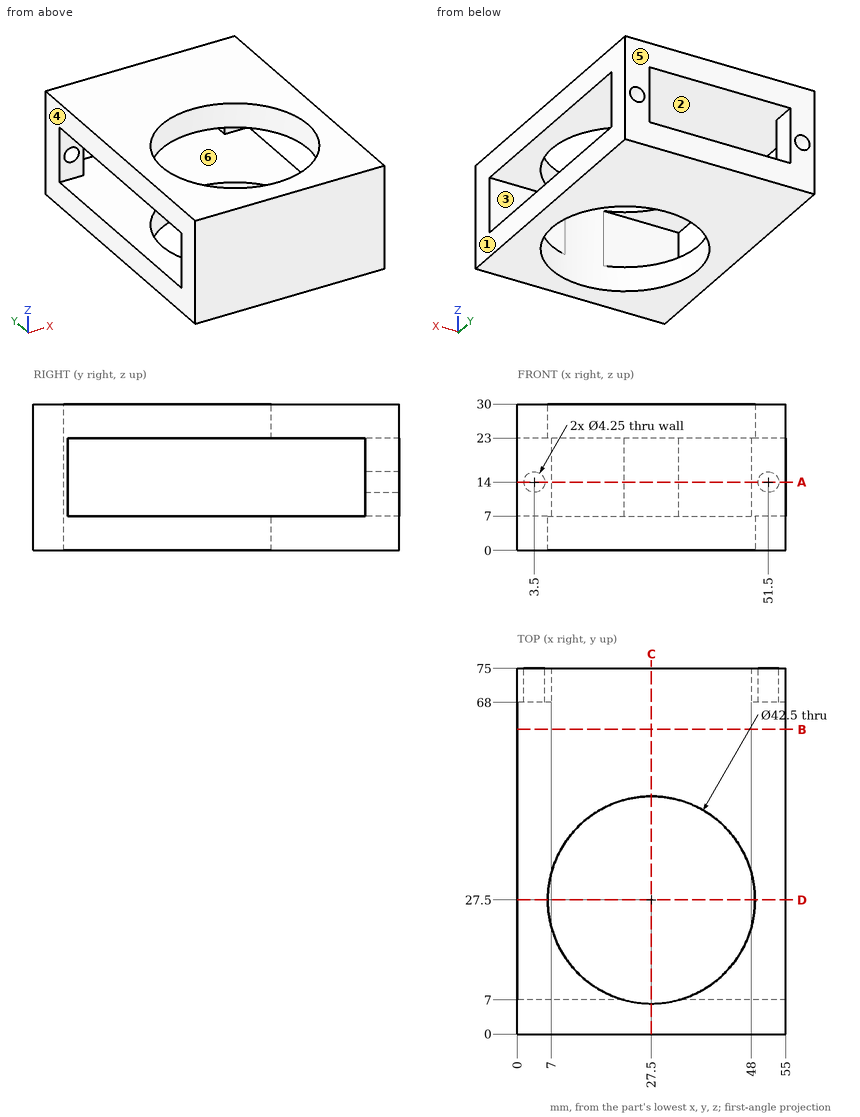
Verification items for this drawing (mm, ordinates from the low corner). A direction names the side the tool comes from. Coordinates: 2 decimals unless noted, no trailing zeros. Order: outer loops, then holes, each group sorted by start corner. A loop starts at its lowest first (then second) coordinate and runs counter-clockwise, first axis right, second up. Notation, with made-up numbers: (-27, 42.5) - (29, 42.5) arc R30 cw to (29, 78.5) - close; hole circle Ø7 at (-38, -34.5). An arc over 180 degrees is marked (long way). Answer as a JSON object with one key per item and string values. Group by question number.
Item 1: Depth check by flat-ended pin: pin 1 Ø3.5 at (x, z) = (3.5, 14) entering from +Y. Enter the tip coordinate at first touch or a pass-through.
Item 2: Sectioned sample at D-D, the plane y = 27.5. Record the cut outline in (x, z).
Item 3: Scan lines: probe 1 along X at (y, z) = (73, 14) (3 decimals); probe 2 along Z at (x, y) = (9.5, 70); probe 3 along Y at (x, z) = (49, 22). Record each from-to range of solid material in increasing order.
Item 4: Draft check along Y on the marked faces 4, 5 and 6. Enter one of: +Y half, -Y half, draft (parallel to the pull), parting line (faces both ways), or undercut.
Item 5: Sectioned sample at B-B, the plane y = 62.5. Record the cut outline in (x, z).
Item 6: Sectioned sample at C-C, the plane x = 27.5. Record the cut outline in (y, z).
Item 7: Tool access check on the marked faces 1, 2 and 3. Record the directions out of +Z, -Z, +X, -X, +Y, -Y that give a thin tool (end or side, any length) a straight path to the whole face; none if there is none.
Item 8: Sectioned sample at A-A, the plane z = 14. Record the cut outline in (x, y) (3 decimals), and give its area (3 significant figures).
Resolved:
{
 "1": {"pin 1": "y = 7"},
 "2": {"outline": "(0, 0) - (6.25, 0) - (6.25, 7) - (0, 7) - close; (0, 23) - (6.25, 23) - (6.25, 30) - (0, 30) - close; (48.75, 0) - (55, 0) - (55, 7) - (48.75, 7) - close; (48.75, 23) - (55, 23) - (55, 30) - (48.75, 30) - close"},
 "3": {"probe 1": "0 to 1.375, 5.625 to 7, 48 to 49.375, 53.625 to 55", "probe 2": "0 to 7, 23 to 30", "probe 3": "0 to 7, 68 to 75"},
 "4": {"face 4": "draft", "face 5": "+Y half", "face 6": "undercut"},
 "5": {"outline": "(0, 0) - (55, 0) - (55, 7) - (0, 7) - close; (0, 23) - (55, 23) - (55, 30) - (0, 30) - close"},
 "6": {"outline": "(0, 0) - (6.25, 0) - (6.25, 30) - (0, 30) - close; (48.75, 0) - (75, 0) - (75, 7) - (48.75, 7) - close; (48.75, 23) - (75, 23) - (75, 30) - (48.75, 30) - close"},
 "7": {"face 1": "+Z, -Z, +X, +Y, -Y", "face 2": "none", "face 3": "+X, -X"},
 "8": {"outline": "(0, 0) - (55, 0) - (55, 7) - (33.096, 7) arc R21.25 cw to (21.904, 7) - (0, 7) - close; (0, 68) - (1.375, 68) - (1.375, 75) - (0, 75) - close; (5.625, 68) - (7, 68) - (7, 75) - (5.625, 75) - close; (48, 68) - (49.375, 68) - (49.375, 75) - (48, 75) - close; (53.625, 68) - (55, 68) - (55, 75) - (53.625, 75) - close", "area": "418 mm^2"}
}
